For this review, take the finished solid that the model builds, in its own axes (mm). A direction names the side the tool comes from. Round coordinates to 2 decimals unless told otherwise and drop trailing zeros. Order: outer loops, then holes, each group sorted by start corner. A loop starts at its lowest first (then second) coordinate and runs counter-clockwise, first axis right, second up. Notation, with made-up numbers: (43.25, 68.25) - (49.25, 68.25) arc R19 cw to (49.25, 103.25) - close; hole circle Ø6 at (58.5, 77). An arc over 180 degrees is marked (long way). One line per item, written item: value.
```python
from build123d import *

# Parameters (mm, degrees)
BASE_FLANGE1_DEPTH          = 102.87
SKETCH6_W                   = 9.525
SKETCH6_H                   = 99.06
CUT_EXTRUDE1_DEPTH          = 10.16
FILLET1_R                   = 21.336
FILLET2_R                   = 12.7
SKETCH8_W                   = 177.8
SKETCH8_H                   = 66.675
CUT_EXTRUDE2_DEPTH          = 10.16
F_27_0_144_DIAMETER_HOLE1_D = 3.6576
F_27_0_144_DIAMETER_HOLE2_D = 3.6576
CUT_EXTRUDE3_REACH          = 210.856
SKETCH17_R                  = 1.6
SKETCH17_W                  = 22.86
SKETCH17_H                  = 17.15
CUT_EXTRUDE4_REACH          = 210.856
SKETCH18_R                  = 5.5499


# Sheet-metal steps are written as plain solids
with BuildPart() as part:
    # Sketch1 → Base-Flange1 (new, symmetric)
    with BuildSketch(Plane.YZ):
        with BuildLine():
            Line((-25.4, -73.66), (-25.4, 15.875))
            ThreePointArc((-25.4, 15.875), (-22.610192091, 22.610192091), (-15.875, 25.4))
            Line((-15.875, 25.4), (152.4, 25.4))
            Line((152.4, 25.4), (152.4, 22.225))
            Line((152.4, 22.225), (-15.875, 22.225))
            ThreePointArc((-15.875, 22.225), (-20.365128061, 20.365128061), (-22.225, 15.875))
            Line((-22.225, 15.875), (-22.225, -73.66))
            Line((-22.225, -73.66), (-25.4, -73.66))
        make_face()
    extrude(amount=BASE_FLANGE1_DEPTH, both=True)

    # Sketch6 → Cut-Extrude1 (cut)
    with BuildSketch(Plane.YZ.offset(102.87)):
        with Locations((-20.6375, -24.13)):
            Rectangle(SKETCH6_W, SKETCH6_H)
    cut_extrude1 = extrude(amount=-CUT_EXTRUDE1_DEPTH, mode=Mode.SUBTRACT)

    # Mirror1: Cut-Extrude1 across plane
    add(cut_extrude1.mirror(Plane(origin=(0, 0, 0), x_dir=(0, 0, 1), z_dir=(1, 0, 0))), mode=Mode.SUBTRACT)

    # Fillet1
    fillet1_edges = [part.edges().sort_by_distance(p)[0] for p in [
        (102.87, 152.4, 23.8125),
        (-102.87, 152.4, 23.8125),
    ]]
    fillet(fillet1_edges, radius=FILLET1_R)

    # Fillet2
    fillet2_edges = [part.edges().sort_by_distance(p)[0] for p in [
        (92.71, -23.8125, -73.66),
        (-92.71, -23.8125, -73.66),
    ]]
    fillet(fillet2_edges, radius=FILLET2_R)

    # Sketch8 → Cut-Extrude2 (cut)
    with BuildSketch(Plane.XY.offset(25.4)):
        with Locations((0, 80.9625)):
            Rectangle(SKETCH8_W, SKETCH8_H)
    extrude(amount=-CUT_EXTRUDE2_DEPTH, mode=Mode.SUBTRACT)

    # #27 (0.144) Diameter Hole1 (through all)
    with Locations(Plane.XY.offset(25.4)):
        with Locations((-76.2, 127), (0, 127), (76.2, 127), (76.2, 34.925), (0, 34.925), (-76.2, 34.925)):
            Hole(F_27_0_144_DIAMETER_HOLE1_D / 2)

    # #27 (0.144) Diameter Hole2 (through all)
    with Locations(Plane.XY.offset(25.4)):
        with Locations((92.4814, 141.7574), (95.4278, 73.533), (95.4278, -25.273), (-95.758, -18.034), (-95.758, 66.294), (-92.3544, 141.351), (3.2512, 144.5768)):
            Hole(F_27_0_144_DIAMETER_HOLE2_D / 2)

    # Sketch17 → Cut-Extrude3 (cut, up to next)
    with BuildSketch(Plane.XY.offset(25.4), mode=Mode.PRIVATE) as cut_extrude3_sk1:
        with Locations((-86.89, 5.4)):
            Circle(SKETCH17_R)
    cut_extrude3_tool1 = extrude(cut_extrude3_sk1.sketch, amount=-CUT_EXTRUDE3_REACH, mode=Mode.PRIVATE) & part.part
    # Sketch17 → Cut-Extrude3 (cut, up to next)
    with BuildSketch(Plane.XY.offset(25.4), mode=Mode.PRIVATE) as cut_extrude3_sk2:
        with Locations((-57.89, 5.4)):
            Circle(SKETCH17_R)
    cut_extrude3_tool2 = extrude(cut_extrude3_sk2.sketch, amount=-CUT_EXTRUDE3_REACH, mode=Mode.PRIVATE) & part.part
    # Sketch17 → Cut-Extrude3 (cut, up to next)
    with BuildSketch(Plane.XY.offset(25.4), mode=Mode.PRIVATE) as cut_extrude3_sk3:
        with Locations((-72.39, 5.4)):
            Rectangle(SKETCH17_W, SKETCH17_H)
    cut_extrude3_tool3 = extrude(cut_extrude3_sk3.sketch, amount=-CUT_EXTRUDE3_REACH, mode=Mode.PRIVATE) & part.part
    add(cut_extrude3_tool1.solids().sort_by_distance((-86.89, 5.4, 25.4))[0], mode=Mode.SUBTRACT)
    add(cut_extrude3_tool2.solids().sort_by_distance((-57.89, 5.4, 25.4))[0], mode=Mode.SUBTRACT)
    add(cut_extrude3_tool3.solids().sort_by_distance((-72.39, 5.4, 25.4))[0], mode=Mode.SUBTRACT)

    # Sketch18 → Cut-Extrude4 (cut, up to next)
    with BuildSketch(Plane.XY.offset(25.4), mode=Mode.PRIVATE) as cut_extrude4_sk1:
        with Locations((-39.37, 5.4)):
            Circle(SKETCH18_R)
    cut_extrude4_tool1 = extrude(cut_extrude4_sk1.sketch, amount=-CUT_EXTRUDE4_REACH, mode=Mode.PRIVATE) & part.part
    add(cut_extrude4_tool1.solids().sort_by_distance((-39.37, 5.4, 25.4))[0], mode=Mode.SUBTRACT)


solid = part.part
```
Item 1: Take a section at D-D (y = -12.5). Write out the cut boundary in (x, z) (3 decimals).
Returned:
outline: (-102.87, 22.225) - (102.87, 22.225) - (102.87, 25.4) - (-102.87, 25.4) - close
Item 2: For P1, Ø6, axis at x = 0, y = 127, coming from the -Z side (3 decimals); P2, Ø10.5, axis at y = -19, z = -10.5, coming from the +X side; P3, Ø1, axis at x = -57.5, z = 12.5, coming from the +Y side (3 decimals), all flat-tipped, find the tip position at first contact; note any pin that passes through.
Returned:
P1: z = 22.225
P2: x = 92.71
P3: y = -22.225
Item 3: Take a section at A-A (x = -11). Write out the cut boundary in (y, z) (3 decimals).
Returned:
outline: (-25.4, -73.66) - (-22.225, -73.66) - (-22.225, 15.875) arc R6.35 cw to (-15.875, 22.225) - (47.625, 22.225) - (47.625, 25.4) - (-15.875, 25.4) arc R9.525 ccw to (-25.4, 15.875) - close; (114.3, 22.225) - (152.4, 22.225) - (152.4, 25.4) - (114.3, 25.4) - close
Item 4: Wall thickness on line 1 (Y direction, x = -86, z = 23) (3 decimals); line 2 (Y direction, x = 41.5, z = 8.5) (3 decimals); line 3 (Z direction, x = 77, y = 44.5) (3 decimals): over which ranges is each line inside the solid? List them lowest first.
Returned:
line 1: -22.196 to 4.07, 6.73 to 47.625, 114.3 to 151.927
line 2: -25.4 to -22.225
line 3: 22.225 to 25.4
Item 5: Take a section at C-C (z = -52.5). Write out the cut boundary in (x, y) (3 decimals).
Returned:
outline: (-92.71, -25.4) - (92.71, -25.4) - (92.71, -22.225) - (-92.71, -22.225) - close
Item 6: The part is to be moulded in two halves that separate along Y. For faces 3 (the cylindrical face through (-34.243, 3.274, 23.835)), 4 (the cylindrical face through (1.3, -22.68, 22.54)), 5 (the cylindrical face through (96.79, 145.98, 23.79)), 6 (the flat face through (92.71, -23, -14)), say which applies: +Y half, -Y half, draft (parallel to the pull), parting line (faces both ways), or undercut.
Returned:
face 3: undercut
face 4: -Y half
face 5: +Y half
face 6: draft
Item 7: Take a section at B-B (y = 110). Write out the cut boundary in (x, z) (3 decimals), plus the area to 3 significant figures.
Returned:
outline: (-102.87, 22.225) - (-88.9, 22.225) - (-88.9, 25.4) - (-102.87, 25.4) - close; (88.9, 22.225) - (102.87, 22.225) - (102.87, 25.4) - (88.9, 25.4) - close
area: 88.7 mm^2
Item 8: Machinability: for faces 1 (the flat face through (1, 32, 22.225)), 2 (the flat face through (1, 30, 25.4)), which of the approach directions +Z, -Z, +X, -X, +Y, -Y give a long, thin tool a straight path to every point of the face, cutting with its end or side? Answer none if there is none.
Returned:
face 1: -Z, +X, -X, +Y
face 2: +Z, +X, -X, +Y, -Y
